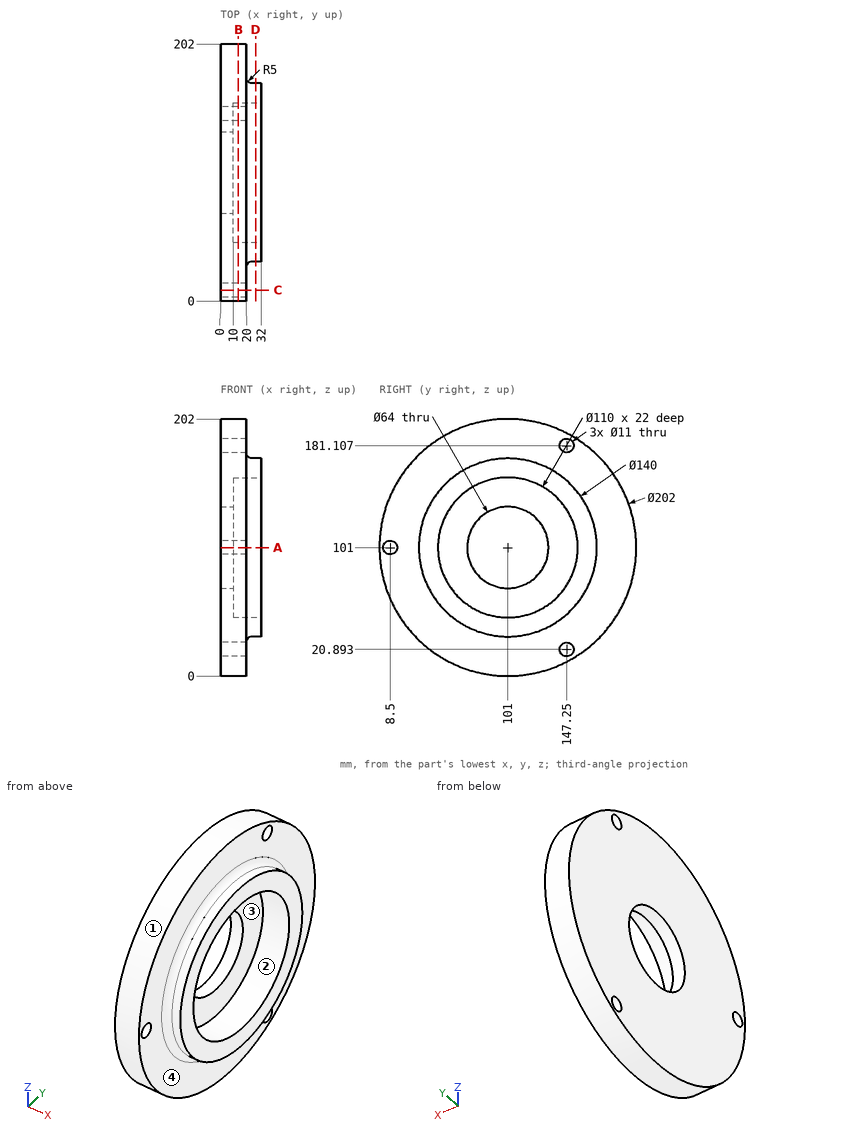
Print and shaded views of the part. All mm, measured from the part's lowest x, y and z. Coordinates: 2 decimals unless noted, no trailing zeros. Loops run counter-clockwise (first coordinate to the right, second up) from the corner with the lowest first, then second, coordinate; pieces in that order, holes last. Notation, with made-up numbers: (39.25, -5) - (49.25, -5) arc R16 ccw to (49.25, 3) - close; hole circle Ø8 at (2.5, 76). An arc over 180 degrees is marked (long way). Write item = value, one per line. Start each with the question number.
Item 1: Drop flat-ended pins along their axis: pin 1 Ø12 at (x, y) = (24.5, 25) entering from -Z; pin 2 Ø9 at (y, z) = (8.5, 101) entering from -X; pin 3 Ø5 at (x, y) = (27.5, 112.5) entering from +Z; pin 4 Ø12.5 at (y, z) = (147.25, 181.11) entering from +X. Give the stop position or say it passes through.
Item 2: Saw through at D-D, the plane x = 27.5. List the corners of the cut face in (y, z), then the cut area to 3 significant figures.
Item 3: Wall check: probe 1 along Z at (x, y) = (8.25, 147.25); probe 2 along X at (y, z) = (51.5, 115); probe 3 along Z at (x, y) = (9, 149) (1 decimal). Give the ranges that are in metal, low to high. Write a range as [from, to].
Item 4: Saw through at B-B, the plane x = 14. List the corners of the cut face in (y, z), then the cut area to 3 significant figures.
Item 5: Saw through at C-C, the plane y = 8.5. List the corners of the cut face in (x, z) (1 decimal), then the cut area to 3 significant figures.
Item 6: Pull direction Y, two halves, no side cores. Call the marked faces 1, 2, 3 and 4: +Y half, -Y half, draft (parallel to the pull), parting line (faces both ways), or undercut.
Item 7: Saw through at A-A, the plane z = 101. List the corners of the cut face in (x, y).
Answers:
q1.pin_1 = 30.2
q1.pin_2 = through
q1.pin_3 = 170.42
q1.pin_4 = 20
q2.outline = circle Ø140 at (101, 101); hole circle Ø110 at (101, 101)
q2.area = 5,890 mm2
q3.probe_1 = [11.21, 15.39], [26.39, 175.61], [186.61, 190.79]
q3.probe_2 = [0, 10]
q3.probe_3 = [12.1, 15.7], [26.1, 175.9], [186.3, 189.9]
q4.outline = circle Ø202 at (101, 101); hole circle Ø11 at (8.5, 101); hole circle Ø110 at (101, 101); hole circle Ø11 at (147.25, 20.89); hole circle Ø11 at (147.25, 181.11)
q4.area = 22,300 mm2
q5.outline = (0, 60.4) - (20, 60.4) - (20, 95.5) - (0, 95.5) - close; (0, 106.5) - (20, 106.5) - (20, 141.6) - (0, 141.6) - close
q5.area = 1,400 mm2
q6.face_1 = parting line
q6.face_2 = undercut
q6.face_3 = undercut
q6.face_4 = draft
q7.outline = (0, 0) - (20, 0) - (20, 3) - (0, 3) - close; (0, 14) - (20, 14) - (20, 26) arc R5 cw to (25, 31) - (32, 31) - (32, 46) - (10, 46) - (10, 69) - (0, 69) - close; (0, 133) - (10, 133) - (10, 156) - (32, 156) - (32, 171) - (25, 171) arc R5 cw to (20, 176) - (20, 202) - (0, 202) - close
